Model file for the job. Use its own axes, mm. Coordinates: 2 decimals unless noted, no trailing zeros. Write each loop counter-clockwise with the first axis right and the second up, starting at its lowest first coordinate (ties: lowest second). Pieces come first, ordered by that corner, then holes. Notation, with made-up numbers: M 0,88.5 L 9,88.5 A16 cw 9,92.5 Z; hole C 38.5,41.5 d10. An arc over 180 degrees is marked long. Put each result on its own line as item: value. Start each with the question number.
Q1. Drop flat-ended pins along their axis: pin 1 (4 mm diameter, centred on x = -50.25, z = 10, fed in from +Y); pin 2 (6 mm diameter, centred on x = -50.25, z = -10, fed in from -Y); pin 3 (1 mm diameter, centred on x = 27.5, y = 1, fed in from -Z). Give the stop position or say it passes through.
Q2. Pull direction Z, two halves, no side cores. Call faces 1 (the cylindrical face through (-49.1, 1.01, -7.78)), 2 (the flat face through (1, 2, 0)), 3 (the cylindrical face through (-102.385, 0.986, -0.751)), 4 (the cylindrical face through (124.994, 0.986, 0.55)): pulls with the +Z half, pulls with the -Z half, needs draft (parallel to the pull), parting line crosses it, or undercut.
Q3. Cut at C-C (x = -50.25). Write the cut outline in (y, z), then the cut area to 3 significant figures.
Q4. Drill centre lines: line 1 along Z through (x, y) = (100, 0.55); line 2 along Z through (x, y) = (-100, 1.5); line 3 along Z through (x, y) = (-25.25, 0.75). Where is each one in solid material? Low to high.
Q5. Cut at A-A (z = 0). Give the number of separate pieces and of enclosed holes in the cut face, then the cut area to 4 significant figures.
Q6. Cut at D-D (x = -112.2). Write the cut outline in (y, z).
```python
from build123d import *

# Parameters (mm, degrees)
BOSS_EXTRUDE1_DEPTH       = 2
F_5_0MM_DOWEL_HOLE1_D     = 5
F_5_0MM_DOWEL_HOLE1_DEPTH = 2
CUT_EXTRUDE1_REACH        = 4
SKETCH4_R                 = 2.5
CUT_EXTRUDE2_REACH        = 4
SKETCH16_R                = 2.5


with BuildPart() as part:
    # Sketch2 → Boss-Extrude1 (new body)
    with BuildSketch(Plane(origin=(0, 0, 0), x_dir=(1, 0, 0), z_dir=(0, 1, 0))):
        with BuildLine():
            Line((100, 25), (-100, 18.75))
            ThreePointArc((-100, 18.75), (-118.75, 0), (-100, -18.75))
            Line((-100, -18.75), (100, -25))
            ThreePointArc((100, -25), (125, 0), (100, 25))
        make_face()
    extrude(amount=BOSS_EXTRUDE1_DEPTH)

    # Ø5.0mm Dowel Hole1
    with Locations(Plane(origin=(0, 2, 0), x_dir=(1, 0, 0), z_dir=(0, 1, 0))):
        with Locations((100, 0), (-100, 0)):
            Hole(F_5_0MM_DOWEL_HOLE1_D / 2, depth=F_5_0MM_DOWEL_HOLE1_DEPTH)

    # Sketch4 → Cut-Extrude1 (cut, up to next)
    with BuildSketch(Plane(origin=(0, 2, 0), x_dir=(1, 0, 0), z_dir=(0, 1, 0)), mode=Mode.PRIVATE) as cut_extrude1_sk1:
        with Locations((100, 12.2)):
            Circle(SKETCH4_R)
    cut_extrude1_tool1 = extrude(cut_extrude1_sk1.sketch, amount=-CUT_EXTRUDE1_REACH, mode=Mode.PRIVATE) & part.part
    add(cut_extrude1_tool1.solids().sort_by_distance((100, 2, -12.2))[0], mode=Mode.SUBTRACT)
    # Sketch4 → Cut-Extrude1 (cut, up to next)
    with BuildSketch(Plane(origin=(0, 2, 0), x_dir=(1, 0, 0), z_dir=(0, 1, 0)), mode=Mode.PRIVATE) as cut_extrude1_sk2:
        with Locations((100, -12.2)):
            Circle(SKETCH4_R)
    cut_extrude1_tool2 = extrude(cut_extrude1_sk2.sketch, amount=-CUT_EXTRUDE1_REACH, mode=Mode.PRIVATE) & part.part
    add(cut_extrude1_tool2.solids().sort_by_distance((100, 2, 12.2))[0], mode=Mode.SUBTRACT)
    # Sketch4 → Cut-Extrude1 (cut, up to next)
    with BuildSketch(Plane(origin=(0, 2, 0), x_dir=(1, 0, 0), z_dir=(0, 1, 0)), mode=Mode.PRIVATE) as cut_extrude1_sk3:
        with Locations((112.2, 0)):
            Circle(SKETCH4_R)
    cut_extrude1_tool3 = extrude(cut_extrude1_sk3.sketch, amount=-CUT_EXTRUDE1_REACH, mode=Mode.PRIVATE) & part.part
    add(cut_extrude1_tool3.solids().sort_by_distance((112.2, 2, 0))[0], mode=Mode.SUBTRACT)
    # Sketch4 → Cut-Extrude1 (cut, up to next)
    with BuildSketch(Plane(origin=(0, 2, 0), x_dir=(1, 0, 0), z_dir=(0, 1, 0)), mode=Mode.PRIVATE) as cut_extrude1_sk4:
        with Locations((87.8, 0)):
            Circle(SKETCH4_R)
    cut_extrude1_tool4 = extrude(cut_extrude1_sk4.sketch, amount=-CUT_EXTRUDE1_REACH, mode=Mode.PRIVATE) & part.part
    add(cut_extrude1_tool4.solids().sort_by_distance((87.8, 2, 0))[0], mode=Mode.SUBTRACT)
    # Sketch4 → Cut-Extrude1 (cut, up to next)
    with BuildSketch(Plane(origin=(0, 2, 0), x_dir=(1, 0, 0), z_dir=(0, 1, 0)), mode=Mode.PRIVATE) as cut_extrude1_sk5:
        with Locations((-100, 12.2)):
            Circle(SKETCH4_R)
    cut_extrude1_tool5 = extrude(cut_extrude1_sk5.sketch, amount=-CUT_EXTRUDE1_REACH, mode=Mode.PRIVATE) & part.part
    add(cut_extrude1_tool5.solids().sort_by_distance((-100, 2, -12.2))[0], mode=Mode.SUBTRACT)
    # Sketch4 → Cut-Extrude1 (cut, up to next)
    with BuildSketch(Plane(origin=(0, 2, 0), x_dir=(1, 0, 0), z_dir=(0, 1, 0)), mode=Mode.PRIVATE) as cut_extrude1_sk6:
        with Locations((-87.8, 0)):
            Circle(SKETCH4_R)
    cut_extrude1_tool6 = extrude(cut_extrude1_sk6.sketch, amount=-CUT_EXTRUDE1_REACH, mode=Mode.PRIVATE) & part.part
    add(cut_extrude1_tool6.solids().sort_by_distance((-87.8, 2, 0))[0], mode=Mode.SUBTRACT)
    # Sketch4 → Cut-Extrude1 (cut, up to next)
    with BuildSketch(Plane(origin=(0, 2, 0), x_dir=(1, 0, 0), z_dir=(0, 1, 0)), mode=Mode.PRIVATE) as cut_extrude1_sk7:
        with Locations((-112.2, 0)):
            Circle(SKETCH4_R)
    cut_extrude1_tool7 = extrude(cut_extrude1_sk7.sketch, amount=-CUT_EXTRUDE1_REACH, mode=Mode.PRIVATE) & part.part
    add(cut_extrude1_tool7.solids().sort_by_distance((-112.2, 2, 0))[0], mode=Mode.SUBTRACT)
    # Sketch4 → Cut-Extrude1 (cut, up to next)
    with BuildSketch(Plane(origin=(0, 2, 0), x_dir=(1, 0, 0), z_dir=(0, 1, 0)), mode=Mode.PRIVATE) as cut_extrude1_sk8:
        with Locations((-100, -12.2)):
            Circle(SKETCH4_R)
    cut_extrude1_tool8 = extrude(cut_extrude1_sk8.sketch, amount=-CUT_EXTRUDE1_REACH, mode=Mode.PRIVATE) & part.part
    add(cut_extrude1_tool8.solids().sort_by_distance((-100, 2, 12.2))[0], mode=Mode.SUBTRACT)

    # Sketch16 → Cut-Extrude2 (cut, up to next)
    with BuildSketch(Plane(origin=(0, 2, 0), x_dir=(1, 0, 0), z_dir=(0, 1, 0)), mode=Mode.PRIVATE) as cut_extrude2_sk1:
        with Locations((-37.749999999, 0)):
            Circle(SKETCH16_R)
    cut_extrude2_tool1 = extrude(cut_extrude2_sk1.sketch, amount=-CUT_EXTRUDE2_REACH, mode=Mode.PRIVATE) & part.part
    add(cut_extrude2_tool1.solids().sort_by_distance((-37.75, 2, 0))[0], mode=Mode.SUBTRACT)
    # Sketch16 → Cut-Extrude2 (cut, up to next)
    with BuildSketch(Plane(origin=(0, 2, 0), x_dir=(1, 0, 0), z_dir=(0, 1, 0)), mode=Mode.PRIVATE) as cut_extrude2_sk2:
        with Locations((-25.249999999, 10)):
            Circle(SKETCH16_R)
    cut_extrude2_tool2 = extrude(cut_extrude2_sk2.sketch, amount=-CUT_EXTRUDE2_REACH, mode=Mode.PRIVATE) & part.part
    add(cut_extrude2_tool2.solids().sort_by_distance((-25.25, 2, -10))[0], mode=Mode.SUBTRACT)
    # Sketch16 → Cut-Extrude2 (cut, up to next)
    with BuildSketch(Plane(origin=(0, 2, 0), x_dir=(1, 0, 0), z_dir=(0, 1, 0)), mode=Mode.PRIVATE) as cut_extrude2_sk3:
        with Locations((-25.249999999, -10)):
            Circle(SKETCH16_R)
    cut_extrude2_tool3 = extrude(cut_extrude2_sk3.sketch, amount=-CUT_EXTRUDE2_REACH, mode=Mode.PRIVATE) & part.part
    add(cut_extrude2_tool3.solids().sort_by_distance((-25.25, 2, 10))[0], mode=Mode.SUBTRACT)
    # Sketch16 → Cut-Extrude2 (cut, up to next)
    with BuildSketch(Plane(origin=(0, 2, 0), x_dir=(1, 0, 0), z_dir=(0, 1, 0)), mode=Mode.PRIVATE) as cut_extrude2_sk4:
        with Locations((-50.249999999, 10)):
            Circle(SKETCH16_R)
    cut_extrude2_tool4 = extrude(cut_extrude2_sk4.sketch, amount=-CUT_EXTRUDE2_REACH, mode=Mode.PRIVATE) & part.part
    add(cut_extrude2_tool4.solids().sort_by_distance((-50.25, 2, -10))[0], mode=Mode.SUBTRACT)
    # Sketch16 → Cut-Extrude2 (cut, up to next)
    with BuildSketch(Plane(origin=(0, 2, 0), x_dir=(1, 0, 0), z_dir=(0, 1, 0)), mode=Mode.PRIVATE) as cut_extrude2_sk5:
        with Locations((-50.249999999, -10)):
            Circle(SKETCH16_R)
    cut_extrude2_tool5 = extrude(cut_extrude2_sk5.sketch, amount=-CUT_EXTRUDE2_REACH, mode=Mode.PRIVATE) & part.part
    add(cut_extrude2_tool5.solids().sort_by_distance((-50.25, 2, 10))[0], mode=Mode.SUBTRACT)


solid = part.part
```
Computed values:
1. pin 1: through
1. pin 2: y = 0
1. pin 3: z = -22.75
2. face 1: undercut
2. face 2: needs draft
2. face 3: undercut
2. face 4: parting line crosses it
3. outline: M 0,-20.3 L 2,-20.3 L 2,-12.5 L 0,-12.5 Z; M 0,-7.5 L 2,-7.5 L 2,7.5 L 0,7.5 Z; M 0,12.5 L 2,12.5 L 2,20.3 L 0,20.3 Z
3. area: 61.2 mm2
4. line 1: -25 to -14.7, -9.7 to -2.5, 2.5 to 9.7, 14.7 to 25
4. line 2: -18.75 to -14.7, -9.7 to -2.5, 2.5 to 9.7, 14.7 to 18.75
4. line 3: -21.09 to -12.5, -7.5 to 7.5, 12.5 to 21.09
5. separate pieces: 8
5. enclosed holes: 0
5. area: 417.5 mm2
6. outline: M 0,-14.24 L 2,-14.24 L 2,-2.5 L 0,-2.5 Z; M 0,2.5 L 2,2.5 L 2,14.24 L 0,14.24 Z
